Read the model definition and answer for the solid it produces. Units are mm, in the model's axes. Face numbers are marked on the shaded views. A direction names the side the tool comes from. Give positions to 0.01 mm unless a question says otherwise; leave off trailing zeros. Write each loop counter-clockwise with the first axis right and the second up, starting at its lowest first coordinate (ties: lowest second). Pieces come first, ordered by that corner, then holes. Notation, with made-up numbers: (58.25, 22.5) -> (104.25, 22.5) arc R8 cw to (104.25, 30.5) -> close; hole circle Ø3 at (42.25, -10). An arc over 180 degrees is marked (long way). Answer as CSV lines item,"result". Start each with the question number.
1. Find the intervals of material crossed by line 1 (Y direction, x = 6.95, z = 7.5); line 2 (Z direction, x = -5.5, y = 0), in increasing order.
2. For a pull along Y with two mould halves and no side action, classify the marked faces 1, 2 and 3 as pulls with the +Y half, pulls with the -Y half, needs draft (parallel to the pull), parting line crosses it, or undercut.
3. The part is cut by section D-D, the plane y = 2.75. Determine the outline of the cut face in (x, z).
4. Given pin 1 (6 mm diameter, centred on y = 0, z = 7.5, fed in from -X); pin 2 (9 mm diameter, centred on x = 0, z = 7.5, fed in from -Y); pin 3 (4 mm diameter, centred on y = 1, z = 7.5, fed in from -X), each flat-ended and moving along its own axis, determine where each tip first touches the part or whether it passes through.
5. The part is cut by section B-B, the plane y = 0. Determine the outline of the cut face in (x, z).
6. The part is cut by section A-A, the plane x = 3. Determine the outline of the cut face in (y, z), and give its area (3 significant figures).
7. A tool of negligible diameter and unlimited length cuts with its end or side. For the marked faces 4, 5, 6, 7 and 8, from which of +Z, -Z, +X, -X, +Y, -Y can it reach the whole face along a straight path? Write none if from no direction.
8. The part is cut by section C-C, the plane z = 7.5. Determine the outline of the cut face in (x, y).
from build123d import *

# Parameters (mm, degrees)
F0_W                 = 15
F0_H                 = 15
F1_DEPTH             = 15
F5_D                 = 5
F5_CBORE_D           = 10
F5_CBORE_DEPTH       = 12
F5_ON_F3_D           = 5
F5_ON_F3_CBORE_D     = 10
F5_ON_F3_CBORE_DEPTH = 12
F5_ON_F4_D           = 5
F5_ON_F4_CBORE_D     = 10
F5_ON_F4_CBORE_DEPTH = 12


with BuildPart() as f1:
    # F0 (on Top) → F1 (new body)
    with BuildSketch(Plane.XY):
        Rectangle(F0_W, F0_H)
    extrude(amount=F1_DEPTH)

    # F5 (through all)
    with Locations(Plane.XZ.offset(7.5)):
        with Locations((0, 7.5)):
            CounterBoreHole(F5_D / 2, F5_CBORE_D / 2, F5_CBORE_DEPTH)

    # F5 on F3 (through all)
    with Locations(Plane(origin=(-7.5, 0, 0), x_dir=(0, -1, 0), z_dir=(-1, 0, 0))):
        with Locations((0, 7.5)):
            CounterBoreHole(F5_ON_F3_D / 2, F5_ON_F3_CBORE_D / 2, F5_ON_F3_CBORE_DEPTH)

    # F5 on F4 (through all)
    with Locations(Plane.XY.offset(15)):
        with Locations((0, 0)):
            CounterBoreHole(F5_ON_F4_D / 2, F5_ON_F4_CBORE_D / 2, F5_ON_F4_CBORE_DEPTH)


solid = f1.part
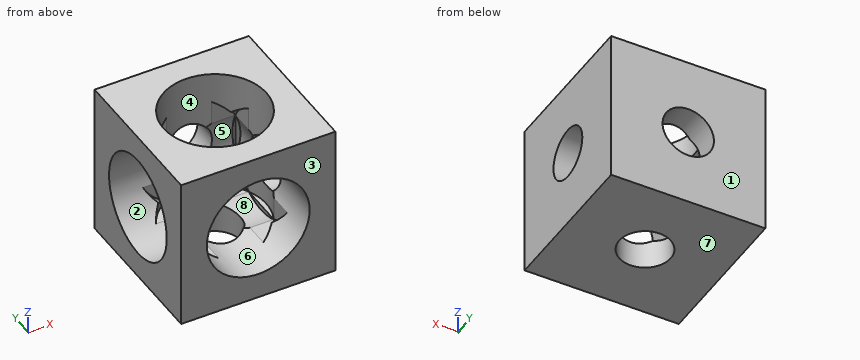
Results found:
1,line 1,"y = -7.5 to -2.5, 2.5 to 7.5"
1,line 2,"z = 0 to 2.5, 12.5 to 15"
2,face 1,"pulls with the +Y half"
2,face 2,"undercut"
2,face 3,"pulls with the -Y half"
3,outline,"(-7.5, 0) -> (7.5, 0) -> (7.5, 15) -> (4.18, 15) -> (4.18, 11.68) -> (4.5, 11.68) -> (4.5, 9.68) arc R5 cw to (4.5, 5.32) -> (4.5, 3.32) -> (4.18, 3.32) -> (4.18, 3) -> (2.18, 3) arc R5 cw to (-2.18, 3) -> (-4.18, 3) -> (-4.18, 3.32) -> (-7.5, 3.32) -> close; (-7.5, 11.68) -> (-4.18, 11.68) -> (-4.18, 15) -> (-7.5, 15) -> close"
4,pin 1,"stops at x = 4.53"
4,pin 2,"stops at y = 4.5"
4,pin 3,"stops at x = 4.66"
5,outline,"(-7.5, 0) -> (-2.5, 0) -> (-2.5, 2.5) -> (-7.5, 2.5) -> close; (-7.5, 12.5) -> (-5, 12.5) -> (-5, 15) -> (-7.5, 15) -> close; (2.5, 0) -> (7.5, 0) -> (7.5, 5) -> (5, 5) -> (5, 3) -> (4.5, 3) -> (4.5, 2.5) -> (2.5, 2.5) -> close; (5, 10) -> (7.5, 10) -> (7.5, 15) -> (5, 15) -> close"
6,outline,"(-7.5, 0) -> (7.5, 0) -> (7.5, 15) -> (4, 15) -> (4, 11.5) -> (4.5, 11.5) -> (4.5, 9.68) arc R5 cw to (4.5, 5.32) -> (4.5, 3.5) -> (4, 3.5) -> (4, 3) -> (2.18, 3) arc R5 cw to (-2.18, 3) -> (-4, 3) -> (-4, 3.5) -> (-7.5, 3.5) -> close; (-7.5, 11.5) -> (-4, 11.5) -> (-4, 15) -> (-7.5, 15) -> close"
6,area,"94.1 mm²"
7,face 4,"+Z"
7,face 5,"-X, -Y"
7,face 6,"-Y"
7,face 7,"-Z, +X, -X, +Y, -Y"
7,face 8,"+Z, -X"
8,outline,"(-7.5, -7.5) -> (-5, -7.5) -> (-5, -5) -> (-7.5, -5) -> close; (-7.5, 5) -> (-2.5, 5) -> (-2.5, 7.5) -> (-7.5, 7.5) -> close; (2.5, 5) -> (4.5, 5) -> (4.5, 4.5) -> (5, 4.5) -> (5, 2.5) -> (7.5, 2.5) -> (7.5, 7.5) -> (2.5, 7.5) -> close; (5, -7.5) -> (7.5, -7.5) -> (7.5, -2.5) -> (5, -2.5) -> close"
